Input: part model. Units: mm. Frame: model coordinates. A direction names the side the tool comes from. Give positions to 0.01 mm unless a question says otherwise; leave off trailing zeros. Write each loop counter-clockwise with the first axis right and the second up, starting at its lowest first coordinate (ties: lowest second). Pieces come first, ordered by that corner, then holes. Notation, with made-up numbers: M 65,53 L 85,53 A14 ccw 85,63 Z; hole C 5.25,65 d2. An arc over 180 degrees is marked long. Use CSV: the item, a comma, the result in double quotes. Start each with the question number.
from build123d import *

# Parameters (mm, degrees)
SKETCH1_R           = 12.7
BOSS_EXTRUDE1_DEPTH = 38.1
SKETCH2_R           = 5.715
CUT_EXTRUDE1_DEPTH  = 43.121134838
SKETCH3_R           = 9.3345
CUT_EXTRUDE2_DEPTH  = 12.7
SKETCH4_R           = 12.7
SKETCH4_R_2         = 5.715
BOSS_EXTRUDE2_DEPTH = 1.27
SKETCH5_W           = 11.43
SKETCH5_H           = 4.572
BOSS_EXTRUDE3_DEPTH = 6.35
BOSS_EXTRUDE4_DEPTH = 4.572
BOSS_EXTRUDE5_START = -39.37
BOSS_EXTRUDE5_DEPTH = 39.37


with BuildPart() as part:
    # Sketch1 → Boss-Extrude1 (new body)
    with BuildSketch(Plane(origin=(0, 0, 0), x_dir=(1, 0, 0), z_dir=(0, 1, 0))):
        with Locations(Location((0, 0, 0), (0, 0, 90))):
            Circle(SKETCH1_R)
    extrude(amount=BOSS_EXTRUDE1_DEPTH)

    # Sketch2 → Cut-Extrude1 (cut, through all)
    with BuildSketch(Plane(origin=(0, 38.1, 0), x_dir=(1, 0, 0), z_dir=(0, 1, 0))):
        with Locations(Location((0, 0, 0), (0, 0, 270))):
            Circle(SKETCH2_R)
    extrude(amount=-CUT_EXTRUDE1_DEPTH, mode=Mode.SUBTRACT)

    # Sketch3 → Cut-Extrude2 (cut)
    with BuildSketch(Plane.XZ):
        with Locations(Location((0, 0, 0), (0, 0, 270))):
            Circle(SKETCH3_R)
    extrude(amount=-CUT_EXTRUDE2_DEPTH, mode=Mode.SUBTRACT)

    # Sketch4 → Boss-Extrude2 (add)
    with BuildSketch(Plane(origin=(0, 38.1, 0), x_dir=(1, 0, 0), z_dir=(0, 1, 0))):
        with Locations(Location((0, 0, 0), (0, 0, 90))):
            Circle(SKETCH4_R)
        with Locations(Location((0, 0, 0), (0, 0, 270))):
            Circle(SKETCH4_R_2, mode=Mode.SUBTRACT)
    extrude(amount=BOSS_EXTRUDE2_DEPTH)

    # Sketch5 → Boss-Extrude3 (add)
    with BuildSketch(Plane(origin=(0, 39.37, 0), x_dir=(1, 0, 0), z_dir=(0, 1, 0))):
        Rectangle(SKETCH5_W, SKETCH5_H)
    extrude(amount=-BOSS_EXTRUDE3_DEPTH)

    # Sketch6 → Boss-Extrude4 (add)
    with BuildSketch(Plane(origin=(0, 0, -2.286), x_dir=(-1, 0, 0), z_dir=(0, 0, -1))):
        Polygon((7.62, 39.37), (-7.62, 39.37), (-3.992504063, 41.91), (3.992504063, 41.91), align=None)
    extrude(amount=-BOSS_EXTRUDE4_DEPTH)

    # Sketch7 → Boss-Extrude5 (add)
    with BuildSketch(Plane(origin=(0, 39.37, 0), x_dir=(1, 0, 0), z_dir=(0, 1, 0)).offset(BOSS_EXTRUDE5_START)):
        with BuildLine():
            ThreePointArc((12.7, 0), (8.980256115, -8.980256127), (-1.7e-08, -12.7))
            Line((-1.7e-08, -12.7), (12.7, -12.7))
            Line((12.7, -12.7), (12.7, 0))
        make_face()
        with BuildLine():
            ThreePointArc((-1.7e-08, -12.7), (-8.980256127, -8.980256115), (-12.7, 0))
            Line((-12.7, 0), (-12.7, -12.7))
            Line((-12.7, -12.7), (-1.7e-08, -12.7))
        make_face()
    extrude(amount=BOSS_EXTRUDE5_DEPTH)


solid = part.part
Q1. Section C-C, the plane y = 8. Return the cut outline in (x, z).
Q2. Set-up query: faces 4 (the cylindrical face through (2.804, 6.261, -8.903)), 5 (the cylindrical face through (0.279, 19.409, -12.697)). Return all of +Z, -Z, +X, -X, +Y, -Y with unobstructed straight access to the full face (end or side cutting, diameter ignored); none if empty.
Q3. Section A-A, the plane y = 37.5. Return the cut outline in (x, z) (3 decimals).
Q4. Material intervals for L1, parallel to Z at x = 0, y = 21 (3 decimals); L2, parallel to Y at x = 10.75, z = 10.5; L3, parallel to Z at x = 8.5, y = 10, sorted ascending. Write a range as [from, to].
Q5. Pull-direction query (Z, two-part tool) for faces 1 (the flat face through (0, 19, 12.7)), 2 (the flat face through (0, 33.02, 0)), 3 (the flat face through (2.6, 39.37, 5.5)); classes: released by +Z, released by -Z, zero draft, split by the parting line, or undercut.
Q6. First-contact query: pin 1 Ø4 at (x, y) = (9, 24) entering from -Z; pin 2 Ø7 at (x, y) = (-1.5, 36) entering from -Z; pin 3 Ø13 at (x, z) = (0, 0) entering from -Y; pin 4 Ø2.5 at (x, z) = (-2.5, 0) entering from -Y. Flat tips, straight axial feed; report the tip coordinate or a pass-through.
Q7. Section B-B, the plane z = 2.75. Return the cut outline in (x, y), and give its area (3 significant figures).
Q8. Section D-D, the plane x = -6.25. Return the cut outline in (y, z), and give its area (3 significant figures).
Check result:
1,outline,"M -12.7,0 A12.7 ccw 12.7,0 L 12.7,12.7 L -12.7,12.7 Z; hole C 0,0 d18.67"
2,face 4,"-Y"
2,face 5,"-Z, +Y, -Y"
3,outline,"M -12.7,0 A12.7 ccw 12.7,0 L 12.7,12.7 L -12.7,12.7 Z; hole M -5.238,-2.286 A5.715 ccw 5.238,-2.286 Z; hole M -5.238,2.286 L 5.238,2.286 A5.715 ccw Z"
4,L1,"z = [-12.7, -5.715], [5.715, 12.7]"
4,L2,"y = [0, 39.37]"
4,L3,"z = [-9.44, -3.86], [3.86, 12.7]"
5,face 1,"released by +Z"
5,face 2,"undercut"
5,face 3,"zero draft"
6,pin 1,"stops at z = -10.6"
6,pin 2,"stops at z = -12.7"
6,pin 3,"stops at y = 12.7"
6,pin 4,"stops at y = 33.02"
7,outline,"M -12.7,0 L -8.92,0 L -8.92,12.7 L -5.01,12.7 L -5.01,39.37 L -12.7,39.37 Z; M 5.01,12.7 L 8.92,12.7 L 8.92,0 L 12.7,0 L 12.7,39.37 L 5.01,39.37 Z"
7,area,"506 mm²"
8,outline,"M 0,-11.06 L 39.37,-11.06 L 39.37,-2.29 L 40.33,-2.29 L 40.33,2.29 L 39.37,2.29 L 39.37,12.7 L 0,12.7 L 0,6.93 L 12.7,6.93 L 12.7,-6.93 L 0,-6.93 Z"
8,area,"764 mm²"
